For this review, use the dimensioned drawing (mm, ordinates from the lowest corner) and the shaded views. Coordinates: 2 decimals unless noted, no trailing zeros. Loops run counter-clockwise (first coordinate to the right, second up) from the corner with the lowest first, then second, coordinate; pieces in that order, holes last. Notation, with made-up numbers: (46, 15) - (64, 15) arc R13 cw to (64, 36) - close; hole circle Ø10 at (2, 16.25). An arc over 180 degrees is marked (long way). Answer in a Markdown table with one row per item. Add a question column.
(1) We need section A-A, the plane y = 251. Write out the cut boundary in (x, z) (1 decimal).
(2) We need section B-B, the plane x = 192. Write out the cut boundary in (y, z) (1 decimal), plus the area to 3 significant figures.
(3) Clearance check with a flat-ended pin moving along its axis: pin 1 (4 mm diameter, centred on x = 289, z = 3, fed in from +Y). State where the tip first meets the part, or that it passes through.
(4) We need section D-D, the plane x = 296.5. Write out the cut boundary in (y, z) (1 decimal).
(5) To check wall thickness, follow L1, parallel to X at y = 254, z = 8.75 (1 decimal); L2, parallel to Y at x = 257.5, z = 9.25 (1 decimal); L3, parallel to Y at x = 302.5, z = 9 (1 decimal). State the ranges of each line that lie inside material, in increasing order. Write a range as [from, to].
(6) The part is to be moulded in two halves that separate along Z. For the marked faces 1 and 2, say which applies: released by +Z, released by -Z, zero draft, split by the parting line, or undercut.
(7) We need section C-C, the plane y = 292.5. Write out the cut boundary in (x, z).
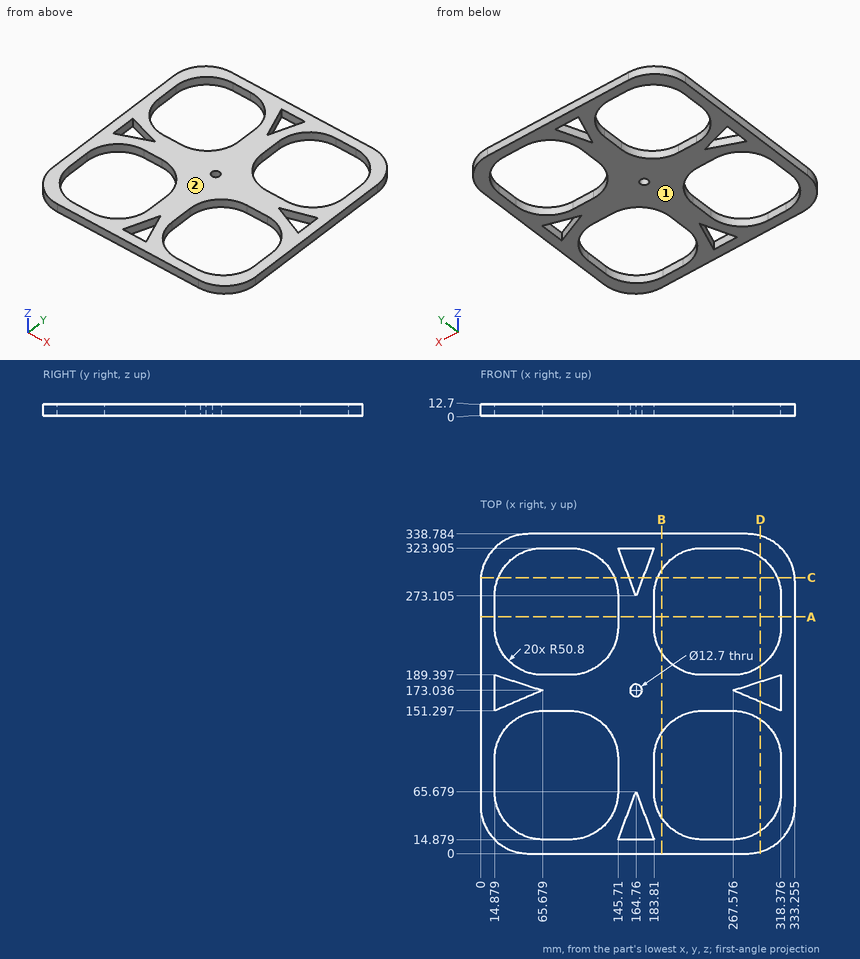
Responses:
| question | item | result |
|---|---|---|
| 1 | outline | (0, 0) - (14.9, 0) - (14.9, 12.7) - (0, 12.7) - close; (145.7, 0) - (183.8, 0) - (183.8, 12.7) - (145.7, 12.7) - close; (318.4, 0) - (333.3, 0) - (333.3, 12.7) - (318.4, 12.7) - close |
| 2 | outline | (0, 0) - (38, 0) - (38, 12.7) - (0, 12.7) - close; (128.2, 0) - (212.5, 0) - (212.5, 12.7) - (128.2, 12.7) - close; (300.8, 0) - (338.8, 0) - (338.8, 12.7) - (300.8, 12.7) - close |
| 2 | area | 2,040 mm2 |
| 3 | pin 1 | stops at y = 338.58 |
| 4 | outline | (2, 0) - (23.9, 0) - (23.9, 12.7) - (2, 12.7) - close; (142.3, 0) - (160.7, 0) - (160.7, 12.7) - (142.3, 12.7) - close; (182.4, 0) - (198.4, 0) - (198.4, 12.7) - (182.4, 12.7) - close; (314.9, 0) - (336.8, 0) - (336.8, 12.7) - (314.9, 12.7) - close |
| 5 | L1 | x = [0, 14.9], [145.7, 183.8], [318.4, 333.3] |
| 5 | L2 | y = [0, 14.9], [151.3, 189.4], [323.9, 338.8] |
| 5 | L3 | y = [4.1, 28.8], [137.4, 158.1], [184.3, 203.3], [310, 334.7] |
| 6 | face 1 | released by -Z |
| 6 | face 2 | released by +Z |
| 7 | outline | (0.2, 0) - (18.73, 0) - (18.73, 12.7) - (0.2, 12.7) - close; (141.86, 0) - (157.49, 0) - (157.49, 12.7) - (141.86, 12.7) - close; (172.03, 0) - (187.66, 0) - (187.66, 12.7) - (172.03, 12.7) - close; (314.53, 0) - (333.05, 0) - (333.05, 12.7) - (314.53, 12.7) - close |
